Source: CAD feature listing. Evaluate the final solid. Frame: model axes, mm. A direction names the side the tool comes from. Round coordinates to 2 decimals unless told otherwise and drop trailing zeros. Write each loop counter-clockwise with the first axis right and the second up, starting at its lowest first coordinate (ties: lowest second). Pieces come first, ordered by that corner, then holes. Notation, with made-up numbers: (84, 77) -> (120, 77) arc R20 cw to (120, 93) -> close; hole circle Ø6 at (3, 54). An arc over 180 degrees is marked (long way). Put each result on its own line as item: value.
```python
from build123d import *

# Parameters (mm, degrees)
PAD041_DEPTH    = 50
SKETCH243_R     = 1.55
POCKET202_DEPTH = 15.001
SKETCH244_R     = 1.55
POCKET203_DEPTH = 10.001


with BuildPart() as part:
    # Sketch242 → Pad041 (new body)
    with BuildSketch(Plane.YZ):
        Polygon((0, 0), (0, 15), (2, 15), (2, 2), (10, 2), (10, 0), align=None)
    extrude(amount=PAD041_DEPTH)

    # Sketch243 (on Face6 of Pad041) → Pocket202 (cut, through all)
    with BuildSketch(Plane.YX):
        with Locations((5, 38)):
            Circle(SKETCH243_R)
        with Locations((5, 12)):
            Circle(SKETCH243_R)
    extrude(amount=-POCKET202_DEPTH, mode=Mode.SUBTRACT)

    # Sketch244 (on Face1 of Pocket202) → Pocket203 (cut, through all)
    with BuildSketch(Plane(origin=(0, 0, 0), x_dir=(0, 0, -1), z_dir=(0, -1, 0))):
        with Locations((-8, 45)):
            Circle(SKETCH244_R)
        with Locations((-8, 5)):
            Circle(SKETCH244_R)
    extrude(amount=-POCKET203_DEPTH, mode=Mode.SUBTRACT)


with BuildPart() as part_1:
    # Body042 placement: moved
    add(part.part.moved(Location((60, -10, 18))))


solid = part_1.part
```
Q1. Cut plane A-A on x = 65. Output: boundary loops of the cut face in (y, z).
Ans:
outline: (-10, 18) -> (0, 18) -> (0, 20) -> (-8, 20) -> (-8, 24.45) -> (-10, 24.45) -> close; (-10, 27.55) -> (-8, 27.55) -> (-8, 33) -> (-10, 33) -> close
Q2. Pin query (flat end, axial travel): pin 1 (5 mm diameter, centred on x = 65, z = 26, fed in from +Y); pin 2 (2.5 mm diameter, centred on x = 91.5, y = -2.5, fed in from +Z). Return the tip coordinate at first contact, or that it passes through.
Ans:
pin 1: stops at y = -8
pin 2: stops at z = 20
Q3. Cut plane B-B on y = -5. Output: boundary loops of the cut face in (x, z), and give its area (3 significant figures).
Ans:
outline: (60, 18) -> (70.45, 18) -> (70.45, 20) -> (60, 20) -> close; (73.55, 18) -> (96.45, 18) -> (96.45, 20) -> (73.55, 20) -> close; (99.55, 18) -> (110, 18) -> (110, 20) -> (99.55, 20) -> close
area: 87.6 mm^2
Q4. Material intervals for line 1 (Z direction, x = 65, y = -8.7); line 2 (X direction, y = -9.3, z = 26); line 3 (Y direction, x = 72, z = 19.2), sorted ascending. Write a range as [from, to].
Ans:
line 1: z = [18, 24.45], [27.55, 33]
line 2: x = [60, 63.45], [66.55, 103.45], [106.55, 110]
line 3: y = [-10, -6.55], [-3.45, 0]
Q5. Reachability of faces 1 (the flat face through (110, -8.3, 23.3)), 2 (the flat face through (85, -8, 27)) from +Z, -Z, +X, -X, +Y, -Y: full face, straight path, thin tool, end or side. Return the list, or none.
Ans:
face 1: +Z, -Z, +X, +Y, -Y
face 2: +Z, +X, -X, +Y
Q6. Draft query along Z for faces 3 (the cylindrical face through (103.487, -9.014, 26.336)), 4 (the cylindrical face through (66.537, -9.014, 26.202)), 5 (the cylindrical face through (99.537, -5.202, 18.986)), 6 (the flat face through (85, -4, 20)). Return one class per face: +Z half, -Z half, draft (parallel to the pull), parting line (faces both ways), or undercut.
Ans:
face 3: undercut
face 4: undercut
face 5: draft
face 6: +Z half
Q7. Cut plane C-C on y = -9.5. Output: boundary loops of the cut face in (x, z).
Ans:
outline: (60, 18) -> (110, 18) -> (110, 33) -> (60, 33) -> close; hole circle Ø3.1 at (65, 26); hole circle Ø3.1 at (105, 26)
Q8. Cut plane D-D on x = 86. Output: boundary loops of the cut face in (y, z), and give its area (3 significant figures).
Ans:
outline: (-10, 18) -> (0, 18) -> (0, 20) -> (-8, 20) -> (-8, 33) -> (-10, 33) -> close
area: 46.0 mm^2
